The listing builds one solid part. Answer for the finished solid, in the listing's coordinates (mm). A direction names the side the tool comes from. Give positions to 0.01 mm unless a question says otherwise; leave off trailing zeros. Loops run counter-clockwise (first coordinate to the right, second up) from the corner with the lowest first, then second, coordinate; pieces in that order, holes last. Notation, with made-up numbers: (-3, 30) - (53, 30) arc R27 ccw to (53, 68) - close; hole circle Ø2 at (84, -3.5). An arc over 180 degrees is marked (long way). Write item = value, one per line. Start each with the question number.
1) A flat-ended cylindrical pin translates along its axis: P1, Ø10, axis at x = -12.5, y = 6.5, coming from the -Z side. Find the tip coordinate at first contact, or state that the pin passes through.
2) The part is cut by section B-B on y = -7. Write down the section's boundary in (x, z).
3) Which of the six approach directions +Z, -Z, +X, -X, +Y, -Y give full straight-line access (tool end or side, diameter ignored) to faces 1 (the flat face through (40.366, 21.639, 0.986)), 2 (the cylindrical face through (-31.585, 17.826, 0.493)), 3 (the cylindrical face through (-32.24, -17.1, 1.49)), 4 (the flat face through (-40.324, 21.639, 0.986)), 5 (the flat face through (32.73, 23.98, 0.49))?
4) The part is cut by section A-A on y = 17. Write down the section's boundary in (x, z).
5) Consider probe 1 along X at (y, z) = (0, 0.25); probe 2 along X at (y, z) = (0.5, 1.4); probe 3 along X at (y, z) = (19, 0.3). Determine where each line is inside the solid, lowest interval first.
6) The part is cut by section D-D on z = 0.35. Write down the section's boundary in (x, y), plus the area to 3 significant figures.
7) The mould has two halves that part along Y. Classify faces 6 (the flat face through (4, -3, 0)), 7 (the cylindrical face through (32.6, 18.07, 1.49)), 8 (the flat face through (-33.594, 23.549, 1.493)), 9 (the cylindrical face through (-32.742, -15.712, 0.493)): +Y half, -Y half, draft (parallel to the pull), parting line (faces both ways), or undercut.
8) The part is cut by section C-C on x = 24. Write down the section's boundary in (y, z), plus the area to 3 significant figures.
from build123d import *
from build123d.topology import SkipClean

# Parameters (mm, degrees)
BASE_EXTRUSION_DEPTH    = 2
ENL_V_START             = -1
ENL_V_MAT_EXTRU_1_DEPTH = 1


with BuildPart() as part:
    # Esquisse1 → Base-Extrusion (new body)
    with BuildSketch(Plane.XY):
        with BuildLine():
            Line((33.747574085, 26.781239692), (31.678333174, 21.096047015))
            ThreePointArc((31.678333174, 21.096047015), (31.641362763, 17.781057074), (33.686188392, 15.171610147))
            ThreePointArc((33.686188392, 15.171610147), (32.319294254, -15.962122137), (6.015631788, 0.75))
            ThreePointArc((6.015631788, 0.75), (4.350969402, 5.153311931), (0.020842383, 7))
            Line((0.020842383, 7), (0.020842383, 3))
            ThreePointArc((0.020842383, 3), (1.464218056, 2.38443731), (2.019105518, 0.916666667))
            ThreePointArc((2.019105518, 0.916666667), (34.168026311, -19.509260389), (35.838674701, 18.543079068))
            ThreePointArc((35.838674701, 18.543079068), (35.429709575, 19.064968454), (35.437103657, 19.727966442))
            Line((35.437103657, 19.727966442), (35.72395853, 20.516093727))
            ThreePointArc((35.72395853, 20.516093727), (36.339050842, 21.119924861), (37.195305146, 21.021035229))
            ThreePointArc((37.195305146, 21.021035229), (37.69827952, 20.696790529), (38.19329026, 20.360513539))
            ThreePointArc((38.19329026, 20.360513539), (38.921758709, 20.193200611), (39.562738511, 20.577654497))
            Line((39.562738511, 20.577654497), (41.19141405, 22.731152258))
            ThreePointArc((41.19141405, 22.731152258), (37.620869006, 25.034414863), (33.747574085, 26.781239692))
        make_face()
    extrude(amount=BASE_EXTRUSION_DEPTH)

    # Esquisse2 → Enlèv. mat.-Extru.1 (cut)
    with BuildSketch(Plane.XY.offset(2).offset(ENL_V_START)):
        with BuildLine():
            Line((33.747574085, 26.781239692), (31.678333174, 21.096047015))
            ThreePointArc((31.678333174, 21.096047015), (31.641362763, 17.781057074), (33.686188392, 15.171610147))
            ThreePointArc((33.686188392, 15.171610147), (32.319294254, -15.962122137), (6.015631788, 0.75))
            ThreePointArc((6.015631788, 0.75), (4.350969402, 5.153311931), (0.020842383, 7))
            Line((0.020842383, 7), (0.020842383, 6))
            ThreePointArc((0.020842383, 6), (3.629281566, 4.461093276), (5.01650022, 0.791666667))
            ThreePointArc((5.01650022, 0.791666667), (32.781477268, -16.8489067), (34.224309969, 16.014477377))
            ThreePointArc((34.224309969, 16.014477377), (32.588449466, 18.102034919), (32.618025795, 20.754026872))
            Line((32.618025795, 20.754026872), (34.681264504, 26.422728636))
            ThreePointArc((34.681264504, 26.422728636), (34.215992075, 26.606080244), (33.747574085, 26.781239692))
        make_face()
    extrude(amount=ENL_V_MAT_EXTRU_1_DEPTH, mode=Mode.SUBTRACT)

    # Bossage-Symétrie1: part across face


with BuildPart() as part_1:
    with SkipClean():  # the faces are left unmerged after this step: merging them gives an invalid solid
        add(part.part)
        add(part.part.mirror(Plane(origin=(0.020842383, 4.785714286, 0.928571429), x_dir=(0, 0, 1), z_dir=(-1, 0, 0))))


solid = part_1.part
Answer below:
q1.P1 = through
q2.outline = (-44.81, 0) - (-40.54, 0) - (-40.54, 1) - (-41.62, 1) - (-41.62, 2) - (-44.81, 2) - close; (-7.38, 0) - (-3.1, 0) - (-3.1, 2) - (-6.29, 2) - (-6.29, 1) - (-7.38, 1) - close; (3.14, 0) - (7.42, 0) - (7.42, 1) - (6.34, 1) - (6.34, 2) - (3.14, 2) - close; (40.58, 0) - (44.86, 0) - (44.86, 2) - (41.66, 2) - (41.66, 1) - (40.58, 1) - close
q3.face_1 = +Z, -Z, +X
q3.face_2 = +Z, -Z
q3.face_3 = +Z
q3.face_4 = +Z, -Z, -X
q3.face_5 = +Z, -Z, +Y
q4.outline = (-37.92, 0) - (-31.94, 0) - (-31.94, 1) - (-33.12, 1) - (-33.12, 2) - (-37.92, 2) - close; (31.98, 0) - (37.96, 0) - (37.96, 2) - (33.17, 2) - (33.17, 1) - (31.98, 1) - close
q5.probe_1 = -45.96 to -41.96, -5.96 to -1.96, 2 to 6, 42 to 46
q5.probe_2 = -45.95 to -42.95, -4.96 to -1.96, 2.01 to 5.01, 42.99 to 45.99
q5.probe_3 = -35.41 to -31.35, 31.39 to 35.45
q6.outline = (-41.15, 22.73) - (-39.52, 20.58) arc R1 ccw to (-38.15, 20.36) arc R24.82 cw to (-37.15, 21.02) arc R1 cw to (-35.68, 20.52) - (-35.4, 19.73) arc R1 cw to (-35.8, 18.54) arc R22 ccw (long way) to (-1.98, 0.92) arc R2 cw (long way) to (2.02, 0.92) arc R22 ccw (long way) to (35.84, 18.54) arc R1 cw to (35.44, 19.73) - (35.72, 20.52) arc R1 cw to (37.2, 21.02) arc R24.82 cw to (38.19, 20.36) arc R1 ccw to (39.56, 20.58) - (41.19, 22.73) arc R28.5 ccw to (33.75, 26.78) - (31.68, 21.1) arc R5 ccw to (33.69, 15.17) arc R18 cw (long way) to (6.02, 0.75) arc R6 ccw (long way) to (-5.97, 0.75) arc R18 cw (long way) to (-33.64, 15.17) arc R5 ccw to (-31.64, 21.1) - (-33.71, 26.78) arc R28.5 ccw to start
q6.area = 831 mm2
q7.face_6 = draft
q7.face_7 = undercut
q7.face_8 = +Y half
q7.face_9 = undercut
q8.outline = (-22, 0) - (-18, 0) - (-18, 1) - (-19, 1) - (-19, 2) - (-22, 2) - close
q8.area = 7.00 mm2
